Here's the drawing with two shaded views (mm, measured from the low corner). I have some questions. Give positions to 0.01 mm unless a question says otherwise; leave off trailing zeros. Loops run counter-clockwise (first coordinate to the right, second up) from the corner with the lowest first, then second, coordinate; pieces in that order, holes last. Notation, with made-up numbers: (-6.75, -6) -> (17.25, -6) arc R29 ccw to (17.25, 17) -> close; hole circle Ø3 at (42, 58). An arc over 180 degrees is marked (long way). Put each result on its own line as item: value.
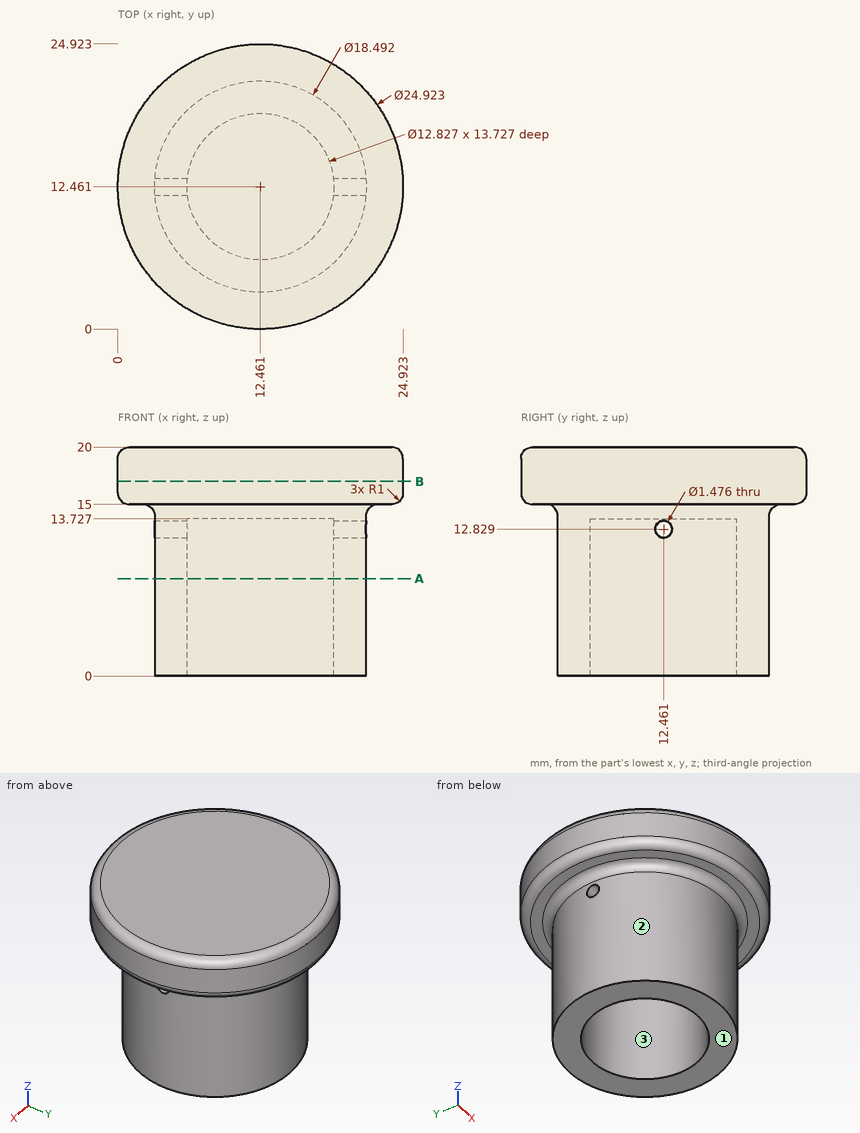
1. If we section it at A-A (z = 8.5): List the corners of the cut face in (x, y) for me (1 decimal), then the cut area to 3 significant figures.
Recorded:
outline: circle Ø18.5 at (12.5, 12.5); hole circle Ø12.8 at (12.5, 12.5)
area: 139 mm^2
2. If we section it at B-B (z = 17): List the corners of the cut face in (x, y) for me.
Recorded:
outline: circle Ø24.92 at (12.46, 12.46)
3. I'm going to push flat-ended pins straight in: pin 1 (7 mm diameter, centred on x = 14, y = 8.5, fed in from -Z); pin 2 (1 mm diameter, centred on x = 15, z = 3, fed in from +Y); pin 3 (10.5 mm diameter, centred on x = 12, y = 12.5, fed in from -Z); pin 4 (1.3 mm diameter, centred on y = 12.46, z = 12.83, fed in from +X). Where does each tip first touch, or does it pass through?
Recorded:
pin 1: stops at z = 0
pin 2: stops at y = 21.48
pin 3: stops at z = 13.73
pin 4: passes through
4. Thinking about a two-plate mould opening in Y: for the marked faces 1, 2 and 3, which applies, pulls with the +Y half, pulls with the -Y half, needs draft (parallel to the pull), parting line crosses it, or undercut?
Recorded:
face 1: needs draft
face 2: parting line crosses it
face 3: undercut
5. I need wall thicknesses on line 1 (Z direction, x = 16, y = 9); line 2 (Y direction, x = 16.5, z = 7) (1 decimal); line 3 (Y direction, x = 20.25, z = 12.5) (1 decimal). Which ranges of each line are inside material? Lowest first, please.
Recorded:
line 1: z = 13.73 to 20
line 2: y = 4.1 to 7.5, 17.4 to 20.8
line 3: y = 7.5 to 11.8, 13.1 to 17.4
